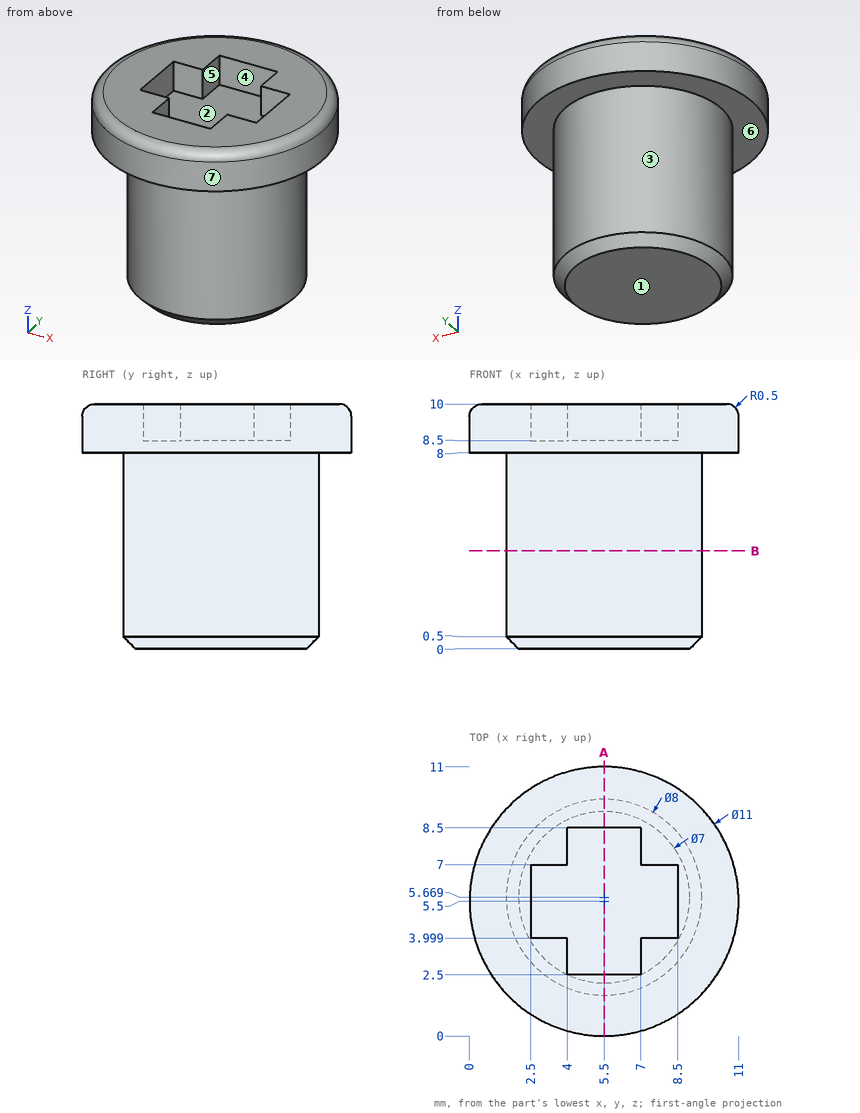
Input: dimensioned drawing with shaded views. Units: mm. Origin: part minimum x, y, z. A direction names the side the tool comes from. Coordinates: 2 decimals unless noted, no trailing zeros. Loops run counter-clockwise (first coordinate to the right, second up) from the corner with the lowest first, then second, coordinate; pieces in that order, holes last. Notation, with made-up numbers: M -29.5,69 L -9.5,69 A19 cw -9.5,85 Z; hole C 70.5,61.5 d8. An arc over 180 degrees is marked long. Use a Markdown table: item, result. Add a question column.
Q1. Section query A-A, the plane x = 5.5. Return loops of the section in (y, z).
Q2. Draft query along X for the marked faces 1, 2, 3 and 4. Return one class per face: pulls with the +X half, pulls with the -X half, needs draft (parallel to the pull), parting line crosses it, or undercut.
Q3. Section query B-B, the plane z = 4. Return loops of the section in (x, y).
Q4. First-contact query: pin 1 (3 mm diameter, centred on y = 9.5, z = 8, fed in from +X); pin 2 (1.2 mm diameter, centred on x = 3, z = 9, fed in from +Y); pin 3 (1 mm diameter, centred on x = 5.5, z = 3.5, fed in from +Y). Flat tips, straight axial feed; report the tip coordinate or a pass-through.
Q5. Access query for the marked faces 5, 6 and 7. Directions: +Z, -Z, +X, -X, +Y, -Y. A direction counts if a zero-diameter tool reaches every point of the face in a straight line with its end or side. Return the directions, or none.
Q6. Material intervals for L1, parallel to Z at x = 9, y = 2; L2, parallel to Z at x = 4.5, y = 5.75; L3, parallel to Y at x = 5.25, z = 6, sorted ascending.
Result:
| question | item | result |
|---|---|---|
| 1 | outline | M 0,8 L 1.67,8 L 1.67,0.5 L 2.17,0 L 9.17,0 L 9.67,0.5 L 9.67,8 L 11,8 L 11,9.5 A0.5 ccw 10.5,10 L 8.5,10 L 8.5,8.5 L 2.5,8.5 L 2.5,10 L 0.5,10 A0.5 ccw 0,9.5 Z |
| 2 | face 1 | needs draft |
| 2 | face 2 | undercut |
| 2 | face 3 | parting line crosses it |
| 2 | face 4 | undercut |
| 3 | outline | C 5.5,5.67 d8 |
| 4 | pin 1 | stops at x = 10.4 |
| 4 | pin 2 | stops at y = 10.66 |
| 4 | pin 3 | stops at y = 9.67 |
| 5 | face 5 | +Z |
| 5 | face 6 | -Z |
| 5 | face 7 | +Z, -Z |
| 6 | L1 | z = 8 to 10 |
| 6 | L2 | z = 0 to 8.5 |
| 6 | L3 | y = 1.68 to 9.66 |
